Could you check a few things on this drawing? It's one solid part, dimensions in mm from its lowest x, y, z. A direction names the side the tool comes from. Give positions to 0.01 mm unless a question says otherwise; leave off trailing zeros. Order: outer loops, then holes, each group sorted by start corner. A loop starts at its lowest first (then second) coordinate and runs counter-clockwise, first axis right, second up. Notation, with made-up numbers: (74, -10.75) -> (95, -10.75) arc R21 cw to (95, 8.25) -> close; hole circle Ø8 at (24, 8.25). An arc over 180 degrees is marked (long way). Write each question's results on one line, items separated by ' | '.
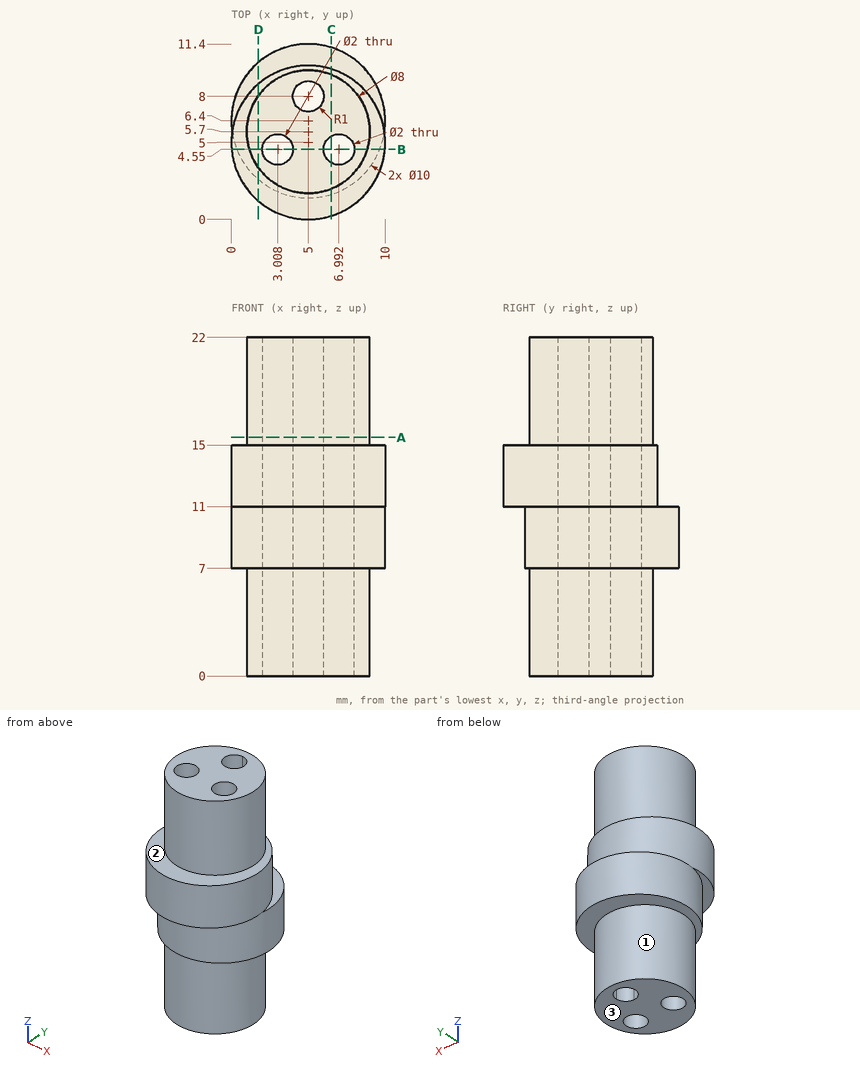
Q1. Suppose I cut it at D-D on x = 1.75. Please give me the cut outline in (y, z).
Here are the results:
outline: (1.2, 11) -> (2.6, 11) -> (2.6, 7) -> (3.37, 7) -> (3.37, 0) -> (8.03, 0) -> (8.03, 7) -> (10.2, 7) -> (10.2, 11) -> (8.8, 11) -> (8.8, 15) -> (8.03, 15) -> (8.03, 22) -> (3.37, 22) -> (3.37, 15) -> (1.2, 15) -> close
Q2. I'm going to push flat-ended pins straight in: pin 1 Ø1 at (x, z) = (8, 8.5) entering from +Y; pin 2 Ø1.5 at (x, z) = (6.5, 10) entering from +Y; pin 3 Ø1.5 at (y, z) = (8, 8.5) entering from +X; pin 4 Ø1.2 at (x, y) = (6.99, 4.55) entering from +Z. Where does each tip first touch, or does it pass through?
Here are the results:
pin 1: stops at y = 10.73 | pin 2: stops at y = 11.34 | pin 3: stops at x = 9.93 | pin 4: passes through
Q3. For the marked faces 1, 2 and 3, which set-ups out of +Z, -Z, +X, -X, +Y, -Y let a thin tool reach every point of the face, with its end or its side?
Here are the results:
face 1: -Z | face 2: +Z | face 3: -Z, +X, -X, +Y, -Y
Q4. I need wall thicknesses on line 1 along Y through (x, z) = (5, 9); line 2 along X through (y, z) = (4.25, 5); line 3 along Y through (x, z) = (5, 4.5). Which ranges of each line are inside material? Lowest first, please.
Here are the results:
line 1: y = 1.4 to 7, 9 to 11.4 | line 2: x = 1.27 to 2.05, 3.96 to 6.04, 7.95 to 8.73 | line 3: y = 1.7 to 7, 9 to 9.7
Q5. Suppose I cut it at C-C on x = 6.5. Please give me the cut outline in (y, z).
Here are the results:
outline: (0.23, 11) -> (1.63, 11) -> (1.63, 7) -> (1.99, 7) -> (1.99, 0) -> (3.68, 0) -> (3.68, 22) -> (1.99, 22) -> (1.99, 15) -> (0.23, 15) -> close; (5.42, 0) -> (9.41, 0) -> (9.41, 7) -> (11.17, 7) -> (11.17, 11) -> (9.77, 11) -> (9.77, 15) -> (9.41, 15) -> (9.41, 22) -> (5.42, 22) -> close
Q6. Suppose I cut it at A-A on z = 15.5. Please give me the cut outline in (x, y).
Here are the results:
outline: circle Ø8 at (5, 5.7); hole circle Ø2 at (3.01, 4.55); hole circle Ø2 at (5, 8); hole circle Ø2 at (6.99, 4.55)
Q7. Suppose I cut it at B-B on y = 4.55. State how many separate pieces and enclosed holes the cut face has.
Here are the results:
separate pieces: 3 | enclosed holes: 0
